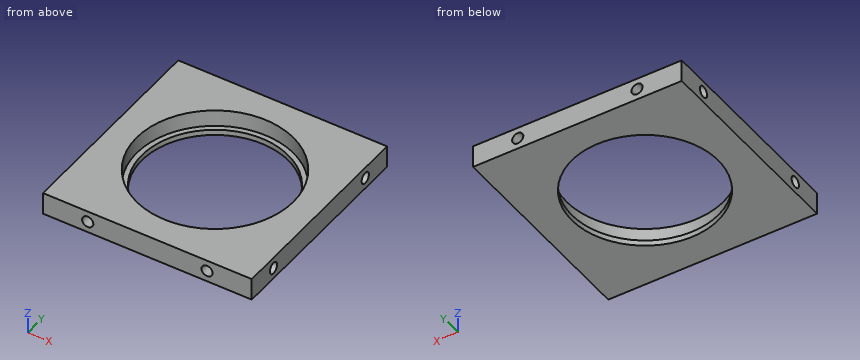
from build123d import *

# Parameters (mm, degrees)
SKETCH_2_W                     = 56
SKETCH_2_H                     = 56
EXTRUDE_1_DEPTH                = 3
M3X0_5_1_D                     = 2.5
M3X0_5_1_DEPTH                 = 8.5
M3X0_5_1_CBORE_D               = 3
M3X0_5_1_CBORE_DEPTH           = 6
M3X0_5_1_TIP                   = 0.751075774
M3X0_5_1_ON_FACE_2_D           = 2.5
M3X0_5_1_ON_FACE_2_DEPTH       = 8.5
M3X0_5_1_ON_FACE_2_CBORE_D     = 3
M3X0_5_1_ON_FACE_2_CBORE_DEPTH = 6
M3X0_5_1_ON_FACE_2_TIP         = 0.751075774
M3X0_5_1_ON_FACE_3_D           = 2.5
M3X0_5_1_ON_FACE_3_DEPTH       = 8.5
M3X0_5_1_ON_FACE_3_CBORE_D     = 3
M3X0_5_1_ON_FACE_3_CBORE_DEPTH = 6
M3X0_5_1_ON_FACE_3_TIP         = 0.751075774
M3X0_5_1_ON_FACE_4_D           = 2.5
M3X0_5_1_ON_FACE_4_DEPTH       = 8.5
M3X0_5_1_ON_FACE_4_CBORE_D     = 3
M3X0_5_1_ON_FACE_4_CBORE_DEPTH = 6
M3X0_5_1_ON_FACE_4_TIP         = 0.751075774


with BuildPart() as part:
    # ｽｹｯﾁ2 → ﾎﾞｽ - 押し出し1 (new, symmetric)
    with BuildSketch(Plane.XY):
        Rectangle(SKETCH_2_W, SKETCH_2_H)
    extrude(amount=EXTRUDE_1_DEPTH, both=True)

    # ｽｹｯﾁ3 → ｶｯﾄ - 回転1 (revolve, cut)
    with BuildSketch(Plane(origin=(0, 0, 0), x_dir=(0, 0, -1), z_dir=(1, 0, 0)), mode=Mode.PRIVATE) as cut_revolve_1_sk:
        Polygon((-3, 21), (1.5, 21), (1.5, 19.61), (3, 19.61), (3, 0), (-3, 0), align=None)
    revolve(cut_revolve_1_sk.sketch.rotate(Axis((0, 0, 0), (0, 0, -1)), 90), axis=Axis((0, 0, 0), (0, 0, -1)), mode=Mode.SUBTRACT)

    # M3x0.5 ねじ穴1
    with Locations(Plane(origin=(-16, 28, 0), x_dir=(1, 0, 0), z_dir=(0, 1, 0))):
        with Locations((0, 0), (32, 0)):
            CounterBoreHole(M3X0_5_1_D / 2, M3X0_5_1_CBORE_D / 2, M3X0_5_1_CBORE_DEPTH, depth=M3X0_5_1_DEPTH)
            with Locations((0, 0, -(M3X0_5_1_DEPTH + M3X0_5_1_TIP / 2))):  # 118° drill point
                Cone(0, M3X0_5_1_D / 2, M3X0_5_1_TIP, mode=Mode.SUBTRACT)

    # M3x0.5 ねじ穴1 on face 2
    with Locations(Plane(origin=(28, 19, 0), x_dir=(0, 0, 1), z_dir=(1, 0, 0))):
        with Locations((0, 0), (0, 38)):
            CounterBoreHole(M3X0_5_1_ON_FACE_2_D / 2, M3X0_5_1_ON_FACE_2_CBORE_D / 2, M3X0_5_1_ON_FACE_2_CBORE_DEPTH, depth=M3X0_5_1_ON_FACE_2_DEPTH)
            with Locations((0, 0, -(M3X0_5_1_ON_FACE_2_DEPTH + M3X0_5_1_ON_FACE_2_TIP / 2))):  # 118° drill point
                Cone(0, M3X0_5_1_ON_FACE_2_D / 2, M3X0_5_1_ON_FACE_2_TIP, mode=Mode.SUBTRACT)

    # M3x0.5 ねじ穴1 on face 3
    with Locations(Plane(origin=(16, -28, 0), x_dir=(0, 0, -1), z_dir=(0, -1, 0))):
        with Locations((0, 0), (0, -32)):
            CounterBoreHole(M3X0_5_1_ON_FACE_3_D / 2, M3X0_5_1_ON_FACE_3_CBORE_D / 2, M3X0_5_1_ON_FACE_3_CBORE_DEPTH, depth=M3X0_5_1_ON_FACE_3_DEPTH)
            with Locations((0, 0, -(M3X0_5_1_ON_FACE_3_DEPTH + M3X0_5_1_ON_FACE_3_TIP / 2))):  # 118° drill point
                Cone(0, M3X0_5_1_ON_FACE_3_D / 2, M3X0_5_1_ON_FACE_3_TIP, mode=Mode.SUBTRACT)

    # M3x0.5 ねじ穴1 on face 4
    with Locations(Plane(origin=(-28, 19, 0), x_dir=(0, 0, -1), z_dir=(-1, 0, 0))):
        with Locations((0, 0), (0, 38)):
            CounterBoreHole(M3X0_5_1_ON_FACE_4_D / 2, M3X0_5_1_ON_FACE_4_CBORE_D / 2, M3X0_5_1_ON_FACE_4_CBORE_DEPTH, depth=M3X0_5_1_ON_FACE_4_DEPTH)
            with Locations((0, 0, -(M3X0_5_1_ON_FACE_4_DEPTH + M3X0_5_1_ON_FACE_4_TIP / 2))):  # 118° drill point
                Cone(0, M3X0_5_1_ON_FACE_4_D / 2, M3X0_5_1_ON_FACE_4_TIP, mode=Mode.SUBTRACT)


solid = part.part
Can you work these out from the model? Positions are in its coordinate system, mm. Round coordinates to 2 decimals unless told otherwise and drop trailing zeros. Write each loop counter-clockwise with the first axis right and the second up, starting at its lowest first coordinate (ties: lowest second). Pieces come first, ordered by that corner, then holes. Notation, with made-up numbers: (-8, 4) - (49, 4) arc R23 cw to (49, 23) - close; hole circle Ø3 at (-38.75, -5.75). An arc over 180 degrees is marked (long way). Write each question's results on one line, items separated by ' | '. Start each with the question number.
1) For pin 1 Ø1.5 at (y, z) = (19, 0) entering from -X; pin 2 Ø1.5 at (x, z) = (-15.5, -0.5) entering from +Y; pin 3 Ø1.5 at (x, z) = (15.5, -0.5) entering from -Y, each with a flat end and sliding along its axis, tell me the tip position at first contact or that it passes through.
2) Suppose I cut it at A-A (y = 0). List the corners of the cut face in (x, z) for me.
3) Suppose I cut it at B-B (x = 0.5). List the corners of the cut face in (y, z) for me.
4) Please list where these lines run through material, in increasing order: line 1 (Y direction, x = -25.9, z = 0); line 2 (Z direction, x = 26, y = 19); line 3 (X direction, y = 4.5, z = 2.6).
Here are the results:
1) pin 1: stops at x = -19.2 | pin 2: stops at y = 22 | pin 3: stops at y = -22
2) outline: (-28, -3) - (-19.61, -3) - (-19.61, -1.5) - (-21, -1.5) - (-21, 3) - (-28, 3) - close; (19.61, -3) - (28, -3) - (28, 3) - (21, 3) - (21, -1.5) - (19.61, -1.5) - close
3) outline: (-28, -3) - (-19.6, -3) - (-19.6, -1.5) - (-20.99, -1.5) - (-20.99, 3) - (-28, 3) - close; (19.6, -3) - (28, -3) - (28, 3) - (20.99, 3) - (20.99, -1.5) - (19.6, -1.5) - close
4) line 1: y = -28 to -20.5, -17.5 to 17.5, 20.5 to 28 | line 2: z = -3 to -1.5, 1.5 to 3 | line 3: x = -28 to -20.51, 20.51 to 28
